Check sheet for the modelled part. Datum: model origin and axes. Units: mm. Face numbers are marked on the shaded views. Coordinates: 2 decimals unless noted, no trailing zeros. Loops run counter-clockwise (first coordinate to the right, second up) from the corner with the lowest first, then second, coordinate; pieces in that order, holes last.
```python
from build123d import *

# Parameters (mm, degrees)
SKETCH_1_R               = 9.9
EXTRUDE_1_DEPTH          = 1.5
SKETCH_2_R               = 1.55
SKETCH_2_W               = 2.5
SKETCH_2_H               = 5
CUT_EXTRUDE_1_DEPTH      = 4
PATTERN_CIRCULAR_1_COUNT = 5
SKETCH_3_R               = 0.6
CUT_EXTRUDE_2_DEPTH      = 4
PATTERN_CIRCULAR_2_COUNT = 5
SKETCH_4_R               = 2.5
CUT_EXTRUDE_3_DEPTH      = 4


with BuildPart() as part:
    # 草图1 → 凸台-拉伸1 (new body, symmetric)
    with BuildSketch(Plane.XY):
        Circle(SKETCH_1_R)
    extrude(amount=EXTRUDE_1_DEPTH, both=True)

    # 草图2 → 切除-拉伸1 (cut, through all)
    with BuildSketch(Plane.XY.offset(1.5)):
        with Locations((0, -6.5)):
            Circle(SKETCH_2_R)
        with Locations((0, 6)):
            Rectangle(SKETCH_2_W, SKETCH_2_H)
    cut_extrude_1 = extrude(amount=-CUT_EXTRUDE_1_DEPTH, mode=Mode.SUBTRACT)

    # 阵列(圆周)1: 切除-拉伸1 ×5 about axis
    pattern_circular_1_axis = Axis((0, 0, 0), (0, 0, 1))
    for i in range(1, PATTERN_CIRCULAR_1_COUNT):
        add(cut_extrude_1.rotate(pattern_circular_1_axis, i * 360 / PATTERN_CIRCULAR_1_COUNT), mode=Mode.SUBTRACT)

    # 草图3 → 切除-拉伸2 (cut, through all)
    with BuildSketch(Plane.XY.offset(1.5)):
        with Locations((1.25, 7.9)):
            Circle(SKETCH_3_R)
        with Locations((-1.25, 7.9)):
            Circle(SKETCH_3_R)
        with Locations((-1.25, 4.1)):
            Circle(SKETCH_3_R)
        with Locations((1.25, 4.1)):
            Circle(SKETCH_3_R)
    cut_extrude_2 = extrude(amount=-CUT_EXTRUDE_2_DEPTH, mode=Mode.SUBTRACT)

    # 阵列(圆周)2: 切除-拉伸2 ×5 about axis
    pattern_circular_2_axis = Axis((0, 0, 0), (0, 0, 1))
    for i in range(1, PATTERN_CIRCULAR_2_COUNT):
        add(cut_extrude_2.rotate(pattern_circular_2_axis, i * 360 / PATTERN_CIRCULAR_2_COUNT), mode=Mode.SUBTRACT)

    # 草图4 → 切除-拉伸3 (cut, through all)
    with BuildSketch(Plane.XY.offset(1.5)):
        Circle(SKETCH_4_R)
    extrude(amount=-CUT_EXTRUDE_3_DEPTH, mode=Mode.SUBTRACT)


solid = part.part
```
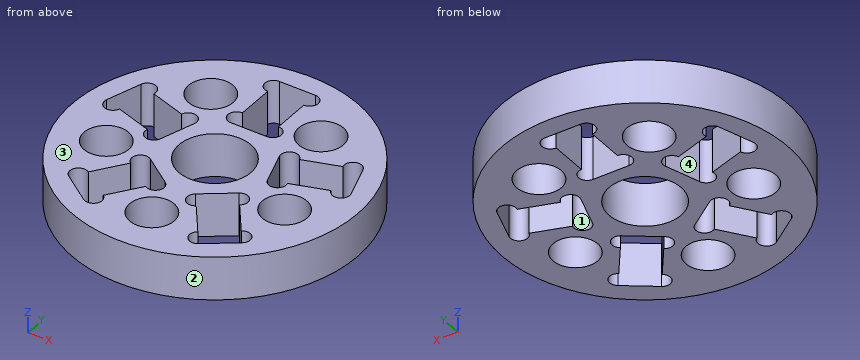
1) Section check B-B on y = -1.25. Enter the section's corners in (x, z), plus the area to 3 significant figures.
Answer sheet:
outline: (-9.82, -1.5) - (-7.53, -1.5) - (-7.53, 1.5) - (-9.82, 1.5) - close; (-4.83, -1.5) - (-2.17, -1.5) - (-2.17, 1.5) - (-4.83, 1.5) - close; (2.17, -1.5) - (4.83, -1.5) - (4.83, 1.5) - (2.17, 1.5) - close; (7.53, -1.5) - (9.82, -1.5) - (9.82, 1.5) - (7.53, 1.5) - close
area: 29.7 mm2
2) Section check C-C on z = 1.1. Give the number of separate pieces and of enclosed holes in the cut face, plus the area to 3 significant figures.
Answer sheet:
separate pieces: 1
enclosed holes: 11
area: 177 mm2
3) Mould release check, pull along X, two halves, no side actions. Record for the marked faces 1, 2, 3 and 4: +X half, -X half, draft (parallel to the pull), parting line (faces both ways), or undercut.
Answer sheet:
face 1: undercut
face 2: parting line
face 3: draft
face 4: undercut
4) Section check A-A on x = 0. Enter the section's corners in (y, z), plus the area to 3 significant figures.
Answer sheet:
outline: (-9.9, -1.5) - (-8.05, -1.5) - (-8.05, 1.5) - (-9.9, 1.5) - close; (-4.95, -1.5) - (-2.5, -1.5) - (-2.5, 1.5) - (-4.95, 1.5) - close; (2.5, -1.5) - (3.5, -1.5) - (3.5, 1.5) - (2.5, 1.5) - close; (8.5, -1.5) - (9.9, -1.5) - (9.9, 1.5) - (8.5, 1.5) - close
area: 20.1 mm2
5) Scan lines: line 1 (Y direction, x = -7, z = 0.7); line 2 (Y direction, x = 0, z = 0.7); line 3 (X direction, y = 5, z = -0.5). Record each from-to range of solid material in increasing order.
Answer sheet:
line 1: y = -7 to -3.33, -0.69 to 0.96, 4.22 to 7
line 2: y = -9.9 to -8.05, -4.95 to -2.5, 2.5 to 3.5, 8.5 to 9.9
line 3: x = -8.54 to -5.35, -2.29 to -1.25, 1.25 to 2.29, 5.35 to 8.54
6) Depth check by flat-ended pin: pin 1 (5 mm diameter, centred on x = 6.18, y = -2.01, fed in from +Z); pin 2 (1.5 mm diameter, centred on y = -4.5, z = -1, fed in from -X); pin 3 (1.5 mm diameter, centred on x = -1.5, z = 1, fed in from -Y); pin 4 (1 mm diameter, centred on y = 5.5, z = 0, fed in from -X). Enter the tip coordinate at first touch or a pass-through.
Answer sheet:
pin 1: stops at z = 1.5
pin 2: stops at x = -9.16
pin 3: stops at y = -9.87
pin 4: stops at x = -8.54
